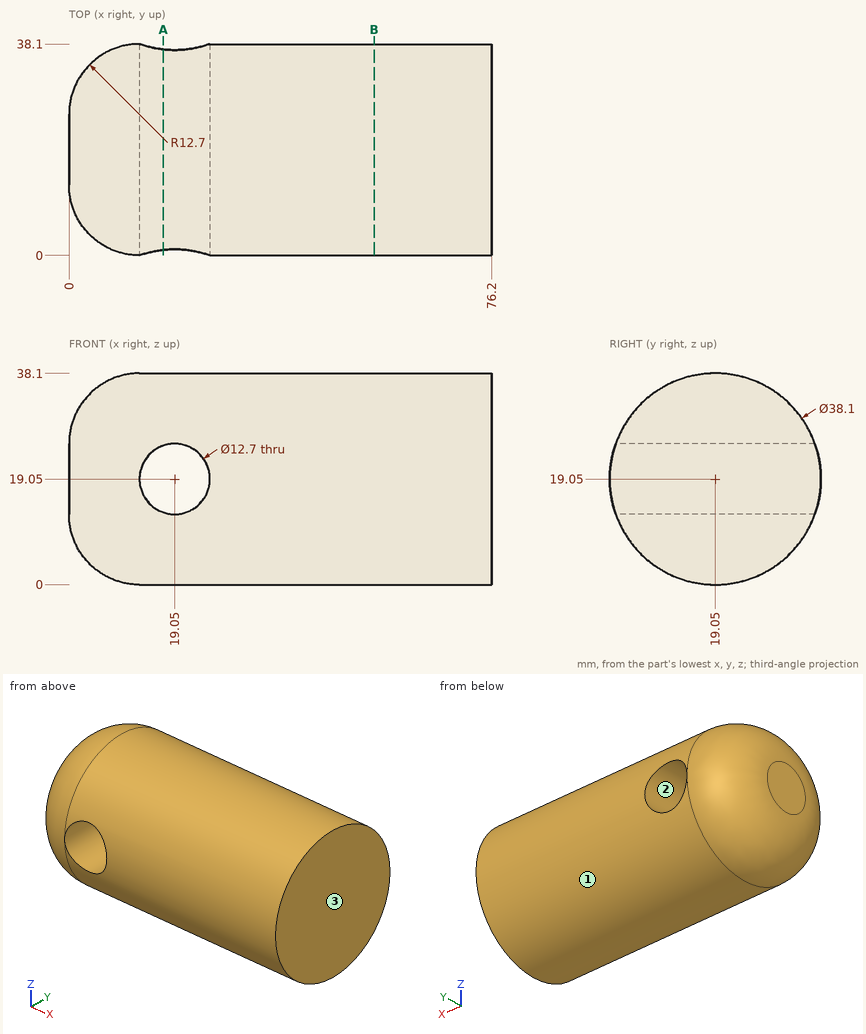
Source: three-view drawing plus pictorial views. Frame: mm from the lowest corner of the part. Round coordinates to 2 decimals unless told otherwise and drop trailing zeros. Loops run counter-clockwise (first coordinate to the right, second up) from the corner with the lowest first, then second, coordinate; pieces in that order, holes last.
Q1. Ray query, line 1 (Z direction, x = 19.05, y = 15.5); line 2 (X direction, y = 28.5, z = 24); line 3 (X direction, y = 12, z = 24). Return the intervals inside material, ascending.
Q2. Section B-B, the plane x = 55. Return loops of the section in (y, z), plus the area to 3 significant figures.
Q3. First-contact query: P1, Ø12, axis at x = 40, y = 24, coming from the +Z side; P2, Ø1.5, axis at x = 17.5, y = 6, coming from the -Z side; P3, Ø10, axis at x = 19.05, z = 19.05, coming from the -Y side; P4, Ø1, axis at x = 38, y = 21, coming from the -Z side. Flat tips, straight axial feed; report the tip coordinate or a pass-through.
Q4. Mould query, pull axis Z, two halves, no side actions, for the marked faces 1, 2 and 3. Classes: pulls with the +Z half, pulls with the -Z half, needs draft (parallel to the pull), parting line crosses it, or undercut.
Q5. Section A-A, the plane x = 17. Return loops of the section in (y, z), plus the area to 3 significant figures.
Solutions:
1. line 1: z = 0.33 to 12.7, 25.4 to 37.77
1. line 2: x = 0.76 to 15.07, 23.03 to 76.2
1. line 3: x = 0.2 to 15.07, 23.03 to 76.2
2. outline: circle Ø38.1 at (19.05, 19.05)
2. area: 1,140 mm2
3. P1: stops at z = 38.1
3. P2: stops at z = 4.5
3. P3: passes through
3. P4: stops at z = 0.06
4. face 1: parting line crosses it
4. face 2: undercut
4. face 3: needs draft
5. outline: (0.97, 13.04) arc R19.05 ccw to (37.13, 13.04) - close; (0.97, 25.06) - (37.13, 25.06) arc R19.05 ccw to start
5. area: 690 mm2
